Geometry check sheet. Reference: drawing and pictorial views, mm from the part's lowest x, y, z. Round coordinates to 2 decimals unless told otherwise and drop trailing zeros. Order: outer loops, then holes, each group sorted by start corner. A loop starts at its lowest first (then second) coordinate and runs counter-clockwise, first axis right, second up.
(1) Depth check by flat-ended pin: pin 1 (5 mm diameter, centred on x = 280, z = 280, fed in from -Y). Enter the tip coordinate at first touch or a pass-through.
(2) Thickness scan on probe 1 along X at (y, z) = (7.25, 280). Record the ranges inside material, lowest first.
(3) Sectioned sample at A-A, the plane x = 20. Enter the section's corners in (y, z), and give its area (3 significant figures).
(4) Sectioned sample at B-B, the plane z = 280. Enter the section's corners in (x, y).
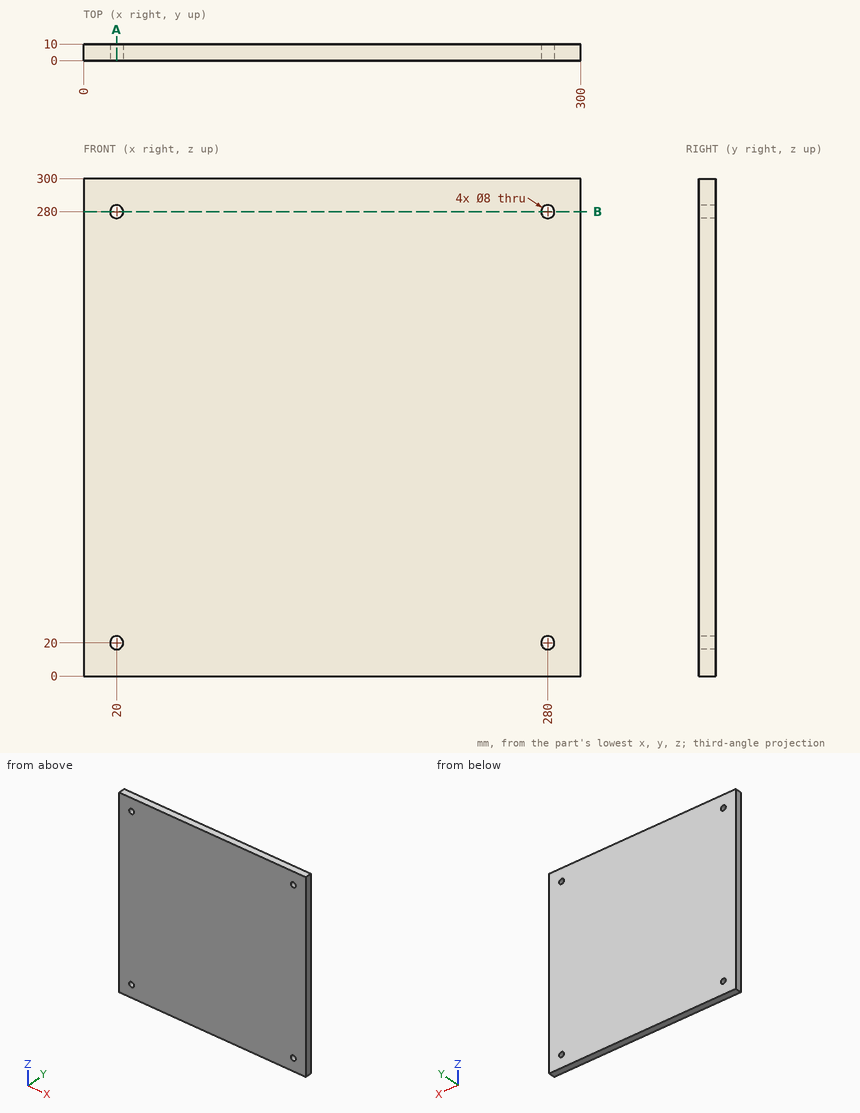
Derived:
1. pin 1: passes through
2. probe 1: x = 0 to 16, 24 to 276, 284 to 300
3. outline: (0, 0) - (10, 0) - (10, 16) - (0, 16) - close; (0, 24) - (10, 24) - (10, 276) - (0, 276) - close; (0, 284) - (10, 284) - (10, 300) - (0, 300) - close
3. area: 2,840 mm2
4. outline: (0, 0) - (16, 0) - (16, 10) - (0, 10) - close; (24, 0) - (276, 0) - (276, 10) - (24, 10) - close; (284, 0) - (300, 0) - (300, 10) - (284, 10) - close
